Verification items for the finished model (mm, model axes). A direction names the side the tool comes from. Coordinates: 2 decimals unless noted, no trailing zeros. Order: outer loops, then holes, each group sorted by start corner. A loop starts at its lowest first (then second) coordinate and runs counter-clockwise, first axis right, second up. Notation, with made-up numbers: M 4,16.5 L 27,16.5 A21 cw 27,35.5 Z; hole C 43.25,29 d3. An arc over 180 degrees is marked long. Return JSON: item names as keys, results as strings. Group by question number.
Q1. Go/stop test with flat-tipped pins: pin 1 Ø12 at (x, z) = (-13.5, -9) entering from +Y; pin 2 Ø0.9 at (x, y) = (-24.5, 5) entering from +Z; pin 3 Ø0.9 at (x, y) = (-25, 4) entering from -Z; pin 4 Ø5 at (x, z) = (-45, -45) entering from -Y. Record where each tip stops, or that it passes through.
Q2. Section check A-A, the plane z = -45. Enter the section's corners in (x, y).
Q3. Section check D-D, the plane y = 0.7. Enter the section's corners in (x, z), then the cut area to 3 significant figures.
Q4. Section check C-C, the plane x = -5. Enter the section's corners in (y, z).
Q5. Thickness scan on probe 1 along Z at (x, y) = (-5, 1.75); probe 2 along X at (y, z) = (1.6, -25); probe 3 along Z at (x, y) = (-43, 0.4). Record the ranges inside material, lowest first.
Q6. Mould release check, pull along Z, two halves, no side actions. Record for faces 6 (the face through (-19, 0, -25)), 7 (the face through (-23.777, 3.042, -22.649)), 8 (the face through (-25, 4, -29)): pulls with the +Z half, pulls with the -Z half, needs draft (parallel to the pull), parting line crosses it, or undercut.
Q7. Section check B-B, the plane x = -25. Enter the section's corners in (y, z).
Q8. Access from +Z, -Z, +X, -X, +Y, -Y to the whole of each face (thin tool, end or side, straight path). Record for faces 1 (the face through (-25, 4, -21)), 2 (the face through (-28.448, 4.479, -22.972)), 3 (the face through (-21.552, 4.479, -27.028)), 4 (the face through (-28.48, 4.48, -26.97)), 5 (the face through (-21.52, 4.48, -23.03)).
Autodesk Inventor part; units mm, degrees
ref_plane "YZ Plane" through (0, 0, 0) normal (1, 0, 0) x (0, 1, 0)
ref_plane "XZ Plane" through (0, 0, 0) normal (0, 1, 0) x (-1, 0, 0)
ref_plane "XY Plane" through (0, 0, 0) normal (0, 0, 1) x (1, 0, 0)
sketch "Sketch1" plane through (0, 0, 0) normal (0, 1, 0) x (-1, 0, 0)
  line L0 (0, 0) -> (50, 0)
  line L1 (50, 0) -> (50, -50)
  line L2 (50, -50) -> (0, -50)
  line L3 (0, -50) -> (0, 0)
  circle A0 centre (45, -5) radius 2.65
  line L4 (50, -25) -> (0, -25)
  line L5 (25, -50) -> (25, 0)
  circle A1 centre (45, -45) radius 2.65
  circle A2 centre (5, -5) radius 2.65
  circle A3 centre (5, -45) radius 2.65
  dimension "d0" = 50
  dimension "d1" = 50
  dimension "d2" = 5
  dimension "d3" = 5
  dimension "d4" = 5.3
extrude "Extrusion1" add sketch "Sketch1" along normal blind 3
sketch "Sketch2" plane through (0, 3, 0) normal (0, 1, 0) x (1, 0, 0)
  line L0 (-20.3812, 25) -> (-22.6906, 21)
  line L1 (-22.6906, 21) -> (-27.3094, 21)
  line L2 (-27.3094, 21) -> (-29.6188, 25)
  line L3 (-29.6188, 25) -> (-27.3094, 29)
  line L4 (-27.3094, 29) -> (-22.6906, 29)
  line L5 (-22.6906, 29) -> (-20.3812, 25)
  line L6 (0, 50) -> (-50, 50)
  line L7 (0, 0) -> (0, 50)
  point P0 (-25, 25)
  point P1 (-25, 21)
  dimension "d7" = 8
  dimension "d8" = 25
  dimension "d9" = 25
extrude "Extrusion2" add sketch "Sketch2" along normal blind 3
sketch "Sketch3" plane through (0, 6, 0) normal (0, 1, 0) x (1, 0, 0)
  circle A0 centre (-25, 25) radius 2.65
  line L0 (0, 50) -> (-50, 50)
  line L1 (0, 0) -> (0, 50)
  dimension "d13" = 5.3
  dimension "d14" = 25
  dimension "d15" = 25
extrude "Extrusion3" cut sketch "Sketch3" against normal blind 10
properties part number "BoxLed"
Numbers:
{
 "1": {"pin 1": "stops at y = 3", "pin 2": "stops at z = -21", "pin 3": "stops at z = -29", "pin 4": "passes through"},
 "2": {"outline": "M -50,0 L -47.65,0 L -47.65,3 L -50,3 Z; M -42.35,0 L -7.65,0 L -7.65,3 L -42.35,3 Z; M -2.35,0 L 0,0 L 0,3 L -2.35,3 Z"},
 "3": {"outline": "M -50,-50 L 0,-50 L 0,0 L -50,0 Z; hole C -45,-45 d5.3; hole C -45,-5 d5.3; hole C -25,-25 d5.3; hole C -5,-45 d5.3; hole C -5,-5 d5.3", "area": "2,390 mm2"},
 "4": {"outline": "M 0,-50 L 3,-50 L 3,-47.65 L 0,-47.65 Z; M 0,-42.35 L 3,-42.35 L 3,-7.65 L 0,-7.65 Z; M 0,-2.35 L 3,-2.35 L 3,0 L 0,0 Z"},
 "5": {"probe 1": "z = -50 to -47.65, -42.35 to -7.65, -2.35 to 0", "probe 2": "x = -50 to -27.65, -22.35 to 0", "probe 3": "z = -50 to -46.74, -43.26 to -6.74, -3.26 to 0"},
 "6": {"face 6": "needs draft", "face 7": "undercut", "face 8": "pulls with the -Z half"},
 "7": {"outline": "M 0,-50 L 3,-50 L 3,-29 L 6,-29 L 6,-27.65 L 0,-27.65 Z; M 0,-22.35 L 6,-22.35 L 6,-21 L 3,-21 L 3,0 L 0,0 Z"},
 "8": {"face 1": "+Z, +X, -X, +Y", "face 2": "+Z, -X, +Y", "face 3": "-Z, +X, +Y", "face 4": "-Z, -X, +Y", "face 5": "+Z, +X, +Y"}
}
